The model under review builds one solid part; all positions refer to its coordinate system, in mm. A direction names the side the tool comes from. Round coordinates to 2 decimals unless told otherwise and drop trailing zeros. Write each loop counter-clockwise with the first axis right and the second up, starting at its lowest first coordinate (ties: lowest second). Pieces come first, ordered by that corner, then holes. Notation, with made-up numbers: (-29.75, -24.5) -> (19.25, -24.5) arc R13 ccw to (19.25, -7.5) -> close; hole circle Ø3 at (-21.75, -35.75). An arc over 180 degrees is marked (long way). Answer as a JSON object with one key per item and string values. Group by question number.
1) Machinability: for faces 1 (the cylindrical face through (-0.04, 18.65, 1.11)), 2 (the flat face through (-1, 0, 0)), which of the approach directions +Z, -Z, +X, -X, +Y, -Y give a long, thin tool a straight path to every point of the face, cutting with its end or side? Answer none if there is none.
2) Insertion check: pin 1 Ø1.5 at (x, y) = (-0.5, 3) entering from -Z. The pin has a flat end and moves straight along its axis. Give the tip position at first contact, or say it passes through.
3) To check wall thickness, follow probe 1 along Y at (x, z) = (0, 0.95). State the ranges of the line that lie inside material, in increasing order. Write a range as [from, to].
4) We need section A-A, the plane x = 0. Write out the cut boundary in (y, z).
5) Mouldability with a two-part tool opening along X and no side actions: class faces 3 (the cylindrical face through (0.04, 22.35, 1.11)), 4 (the flat face through (-8.5, 0, 1)), 5 (the flat face through (-1, -24.5, 1)) as pulls with the +X half, pulls with the -X half, needs draft (parallel to the pull), parting line crosses it, or undercut.
6) We need section B-B, the plane z = 1.35. Write out the cut boundary in (x, y), then the cut area to 3 significant figures.
from build123d import *

# Parameters (mm, degrees)
F0_W    = 15
F0_H    = 49
F0_R    = 1.6
F3_SIZE = 0.2


with BuildPart() as f2:
    # F2: sweep along a path in F1
    with BuildLine(Plane.XZ) as f2_path:
        Line((0, 0), (0, 2))
    # F0 (on Top) → F2 (sweep)
    with BuildSketch(Plane.XY):
        with Locations((-1, 0)):
            Rectangle(F0_W, F0_H)
        with Locations((0, -20.5)):
            Circle(F0_R, mode=Mode.SUBTRACT)
        with BuildLine():
            Line((-1.6, 20.25), (-1.6, 20.75))
            ThreePointArc((-1.6, 20.75), (0, 22.35), (1.6, 20.75))
            Line((1.6, 20.75), (1.6, 20.25))
            ThreePointArc((1.6, 20.25), (0, 18.65), (-1.6, 20.25))
        make_face(mode=Mode.SUBTRACT)
    sweep(path=f2_path.line)

    # F3
    f3_edges = [f2.edges().sort_by_distance(p)[0] for p in [
        (6.5, 0, 0),
        (-1, -24.5, 0),
        (-1, 24.5, 0),
        (-8.5, 0, 0),
        (-1.6, -20.5, 0),
        (0, 18.65, 0),
        (1.6, 20.5, 0),
        (0, 22.35, 0),
        (-1.6, 20.5, 0),
    ]]
    chamfer(f3_edges, length=F3_SIZE)


solid = f2.part
Here are the results:
{
 "1": {"face 1": "+Z, -Z", "face 2": "-Z, +X, -X, +Y, -Y"},
 "2": {"pin 1": "stops at z = 0"},
 "3": {"probe 1": "y = [-24.5, -22.1], [-18.9, 18.65], [22.35, 24.5]"},
 "4": {"outline": "(-24.5, 0.2) -> (-24.3, 0) -> (-22.3, 0) -> (-22.1, 0.2) -> (-22.1, 2) -> (-24.5, 2) -> close; (-18.9, 0.2) -> (-18.7, 0) -> (18.45, 0) -> (18.65, 0.2) -> (18.65, 2) -> (-18.9, 2) -> close; (22.35, 0.2) -> (22.55, 0) -> (24.3, 0) -> (24.5, 0.2) -> (24.5, 2) -> (22.35, 2) -> close"},
 "5": {"face 3": "undercut", "face 4": "pulls with the -X half", "face 5": "needs draft"},
 "6": {"outline": "(-8.5, -24.5) -> (6.5, -24.5) -> (6.5, 24.5) -> (-8.5, 24.5) -> close; hole circle Ø3.2 at (0, -20.5); hole (-1.6, 20.25) arc R1.6 ccw to (1.6, 20.25) -> (1.6, 20.75) arc R1.6 ccw to (-1.6, 20.75) -> close", "area": "717 mm^2"}
}
